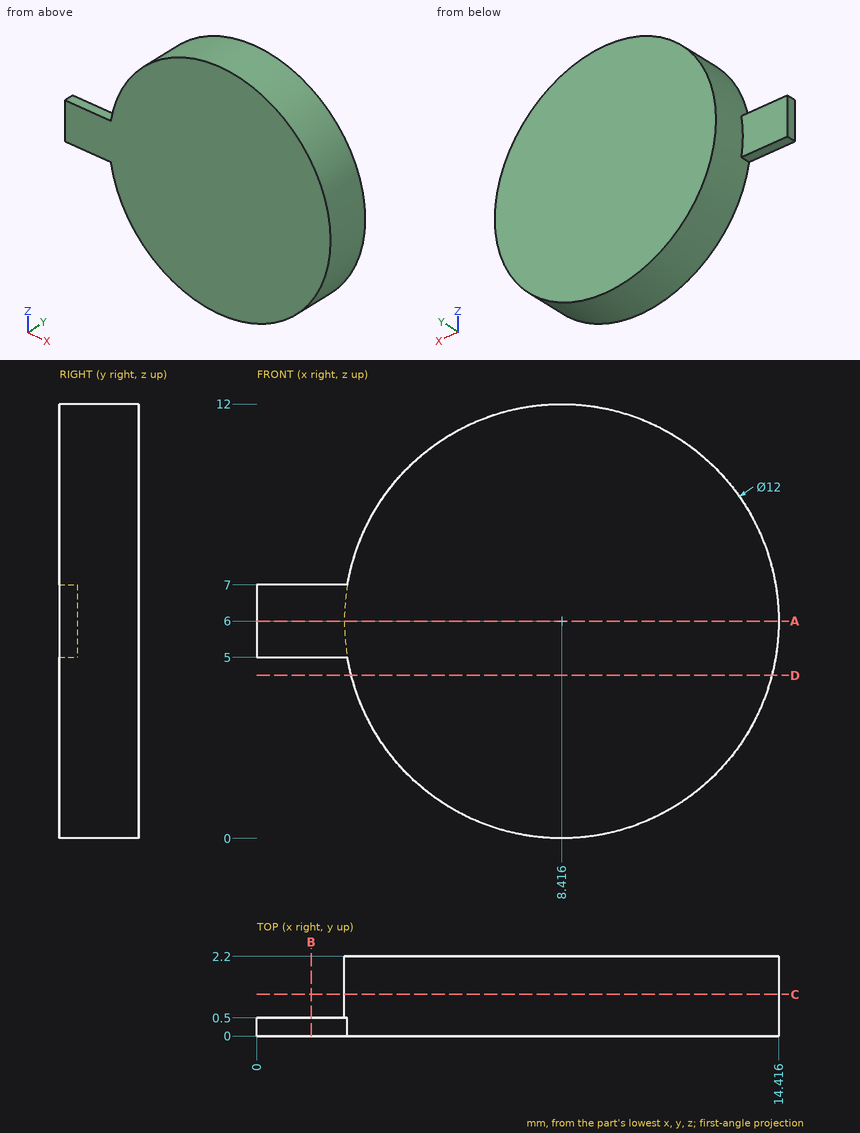
Answer from the drawing. Dimensions are ordinates in mm from the lowest x, y and z of the part. Coordinates: 2 decimals unless noted, no trailing zeros. Loops run counter-clockwise (first coordinate to the right, second up) from the corner with the lowest first, then second, coordinate; pieces in that order, holes last. Notation, with made-up numbers: (77.25, -39) - (116.25, -39) arc R23 cw to (116.25, -18) - close; hole circle Ø6 at (45.25, -7.75). An arc over 180 degrees is marked (long way). Use a Markdown table: item, result.
Item 1: Find section B-B, the plane x = 1.5. Determine the outline of the cut face in (y, z).
Evaluation:
| item | result |
|---|---|
| outline | (0, 5) - (0.5, 5) - (0.5, 7) - (0, 7) - close |
Item 2: Find section C-C, the plane y = 1.15. Determine the outline of the cut face in (x, z), and give its area (3 significant figures).
Evaluation:
| item | result |
|---|---|
| outline | circle Ø12 at (8.42, 6) |
| area | 113 mm2 |
Item 3: Find section A-A, the plane z = 6. Determine the outline of the cut face in (x, y).
Evaluation:
| item | result |
|---|---|
| outline | (0, 0) - (14.42, 0) - (14.42, 2.2) - (2.42, 2.2) - (2.42, 0.5) - (0, 0.5) - close |
Item 4: Consider probe 1 along X at (y, z) = (0.85, 9); probe 2 along X at (y, z) = (0.45, 9.75); probe 3 along Z at (x, y) = (10, 0.8). Determine where each line is inside the solid, lowest interval first. Write a range as from..to.
Evaluation:
| item | result |
|---|---|
| probe 1 | x = 3.22..13.61 |
| probe 2 | x = 3.73..13.1 |
| probe 3 | z = 0.21..11.79 |
Item 5: Find section D-D, the plane z = 4.5. Determine the outline of the cut face in (x, y), and give its area (3 significant figures).
Evaluation:
| item | result |
|---|---|
| outline | (2.61, 0) - (14.23, 0) - (14.23, 2.2) - (2.61, 2.2) - close |
| area | 25.6 mm2 |
Item 6: Given pin 1 Ø0.6 at (x, z) = (2, 5.5) entering from +Y; pin 2 Ø1 at (x, y) = (6, 1.5) entering from -Z; pin 3 Ø0.6 at (x, y) = (1.5, 0.5) entering from +Z, each flat-ended and moving along its own axis, determine where each tip first touches the part or whether it passes through.
Evaluation:
| item | result |
|---|---|
| pin 1 | stops at y = 0.5 |
| pin 2 | stops at z = 0.31 |
| pin 3 | stops at z = 7 |
